CAD build for the part. Positions are in the model's coordinates, mm. A direction names the side the tool comes from. Round coordinates to 2 decimals unless told otherwise and drop trailing zeros. Loops run counter-clockwise (first coordinate to the right, second up) from the corner with the lowest first, then second, coordinate; pieces in that order, holes last. Notation, with made-up numbers: (6.5, 5) -> (54.5, 5) arc R16 ccw to (54.5, 22) -> close; hole circle Ø4 at (65.5, 30.5). An arc over 180 degrees is marked (long way). Answer as CSV lines item,"result".
```python
from build123d import *

# Parameters (mm, degrees)
SKETCH3_R           = 4.075
BOSS_EXTRUDE3_DEPTH = 50
CUT_EXTRUDE1_DEPTH  = 40
SKETCH8_R           = 6
SKETCH8_R_2         = 17.5
CUT_EXTRUDE2_DEPTH  = 6
SKETCH9_R           = 9
SKETCH9_R_2         = 6
BOSS_EXTRUDE4_DEPTH = 30


with BuildPart() as part:
    # Sketch3 → Boss-Extrude3 (new body)
    with BuildSketch(Plane.XY):
        with BuildLine():
            Line((0, 0), (0, 25))
            ThreePointArc((0, 25), (4.917135927, 33.725327913), (14.927715135, 34.038180658))
            Line((14.927715135, 34.038180658), (80, 0))
            Line((80, 0), (80, -5))
            Line((80, -5), (0, -5))
            Line((0, -5), (0, 0))
        make_face()
        with Locations((10.2, 25)):
            Circle(SKETCH3_R, mode=Mode.SUBTRACT)
    extrude(amount=BOSS_EXTRUDE3_DEPTH)

    # Sketch6 → Cut-Extrude1 (cut)
    with BuildSketch(Plane.XY.offset(45)):
        with BuildLine():
            Line((0, 25), (0, 0))
            Line((0, 0), (80, 0))
            Line((80, 0), (14.927715135, 34.038180658))
            ThreePointArc((14.927715135, 34.038180658), (4.917135927, 33.725327913), (0, 25))
        make_face()
    extrude(amount=-CUT_EXTRUDE1_DEPTH, mode=Mode.SUBTRACT)

    # Sketch8 → Cut-Extrude2 (cut, through all)
    with BuildSketch(Plane(origin=(0, 0, 0), x_dir=(1, 0, 0), z_dir=(0, 1, 0))):
        with Locations((10.2, -25)):
            Circle(SKETCH8_R)
        with Locations((50.2, -25)):
            Circle(SKETCH8_R_2)
    extrude(amount=-CUT_EXTRUDE2_DEPTH, mode=Mode.SUBTRACT)

    # Sketch9 → Boss-Extrude4 (add)
    with BuildSketch(Plane(origin=(0, 0, 0), x_dir=(1, 0, 0), z_dir=(0, 1, 0))):
        with Locations((10.2, -25)):
            Circle(SKETCH9_R)
        with Locations((10.2, -25)):
            Circle(SKETCH9_R_2, mode=Mode.SUBTRACT)
    extrude(amount=BOSS_EXTRUDE4_DEPTH)


solid = part.part
```
Q1. Tool access for faces 5 (the cylindrical face through (18.784, 14.79, 22.297)), 6 (the flat face through (32, 11, 50)), 7 (the flat face through (31, 14, 5)): list every direction of +Z, -Z, +X, -X, +Y, -Y with a clear straight run to the whole face (end or side of a thin tool).
Results:
face 5,"+Y"
face 6,"+Z, +X, -X, +Y, -Y"
face 7,"+X, -X, +Y"
Q2. Slice it at A-A, the plane y = 2.5. Give the cut face in (x, z), and give its area (3 significant figures).
Results:
outline,"(0, 0) -> (75.22, 0) -> (75.22, 5) -> (0, 5) -> close; (0, 45) -> (75.22, 45) -> (75.22, 50) -> (0, 50) -> close; circle Ø18 at (10.2, 25); hole circle Ø12 at (10.2, 25)"
area,"894 mm2"
Q3. Two-plate mould, pull along X, no slides. Class faces 1 (the flat face through (32, 11, 0)), 2 (the flat face through (47.008, 17.257, 47.465)), 3 (the cylindrical face through (12.391, 28.436, 47.465)), 4 (the cylindrical face through (12.391, 28.436, 2.465)): pulls with the +X half, pulls with the -X half, needs draft (parallel to the pull), parting line crosses it, or undercut.
Results:
face 1,"needs draft"
face 2,"pulls with the +X half"
face 3,"undercut"
face 4,"undercut"
Q4. Slice it at C-C, the plane z = 25. Give the cut face in (x, y), and give its area (3 significant figures).
Results:
outline,"(0, -5) -> (4.2, -5) -> (4.2, 30) -> (1.2, 30) -> (1.2, 0) -> (0, 0) -> close; (16.2, -5) -> (32.7, -5) -> (32.7, 0) -> (19.2, 0) -> (19.2, 30) -> (16.2, 30) -> close; (67.7, -5) -> (80, -5) -> (80, 0) -> (67.7, 0) -> close"
area,"345 mm2"
Q5. Slice it at B-B, the plane x = 10.2. Give the cut face in (y, z) (3 decimals).
Results:
outline,"(-5, 0) -> (20.925, 0) -> (20.925, 5) -> (0, 5) -> (0, 16) -> (30, 16) -> (30, 19) -> (-5, 19) -> close; (-5, 31) -> (30, 31) -> (30, 34) -> (0, 34) -> (0, 45) -> (20.925, 45) -> (20.925, 50) -> (-5, 50) -> close; (29.075, 0) -> (35.2, 0) -> (35.2, 5) -> (29.075, 5) -> close; (29.075, 45) -> (35.2, 45) -> (35.2, 50) -> (29.075, 50) -> close"
Q6. Probe L1, parallel to X at y = -2.55, z = 25; L2, parallel to Z at x = 27, y = 18; L3, parallel to Z at x = 10.2, y = 12.25. List the from-to ranges inside material, lowest first. Write a range as [from, to].
Results:
L1,"[0, 4.2], [16.2, 32.7], [67.7, 80]"
L2,"[0, 5], [45, 50]"
L3,"[0, 5], [16, 19], [31, 34], [45, 50]"
Q7. Slice it at D-D, the plane y = 22. Give the cut face in (x, z).
Results:
outline,"(0, 0) -> (7.44, 0) -> (7.44, 5) -> (0, 5) -> close; (0, 45) -> (7.44, 45) -> (7.44, 50) -> (0, 50) -> close; circle Ø18 at (10.2, 25); (12.96, 0) -> (37.94, 0) -> (37.94, 5) -> (12.96, 5) -> close; (12.96, 45) -> (37.94, 45) -> (37.94, 50) -> (12.96, 50) -> close; hole circle Ø12 at (10.2, 25)"
Q8. Drop flat-ended pins along their axis: pin 1 Ø19 at (x, z) = (10.2, 25) entering from +Y; pin 2 Ø6.5 at (x, y) = (10.2, 25) entering from +Z; pin 3 Ø10 at (y, z) = (9.5, 25.5) entering from +X. Give the stop position or say it passes through.
Results:
pin 1,"y = 30"
pin 2,"z = 34"
pin 3,"x = 19.2"
